Source: three-view drawing plus pictorial views. Frame: mm from the lowest corner of the part. A direction names the side the tool comes from. Coordinates: 2 decimals unless noted, no trailing zeros. Order: outer loops, then holes, each group sorted by start corner. A loop starts at its lowest first (then second) coordinate and runs counter-clockwise, first axis right, second up. Notation, with made-up numbers: M 23.5,60 L 73.5,60 A19 ccw 73.5,79 Z; hole C 11.5,22.25 d11. An arc over 180 degrees is marked long. One line per question, with ' | ' between items.
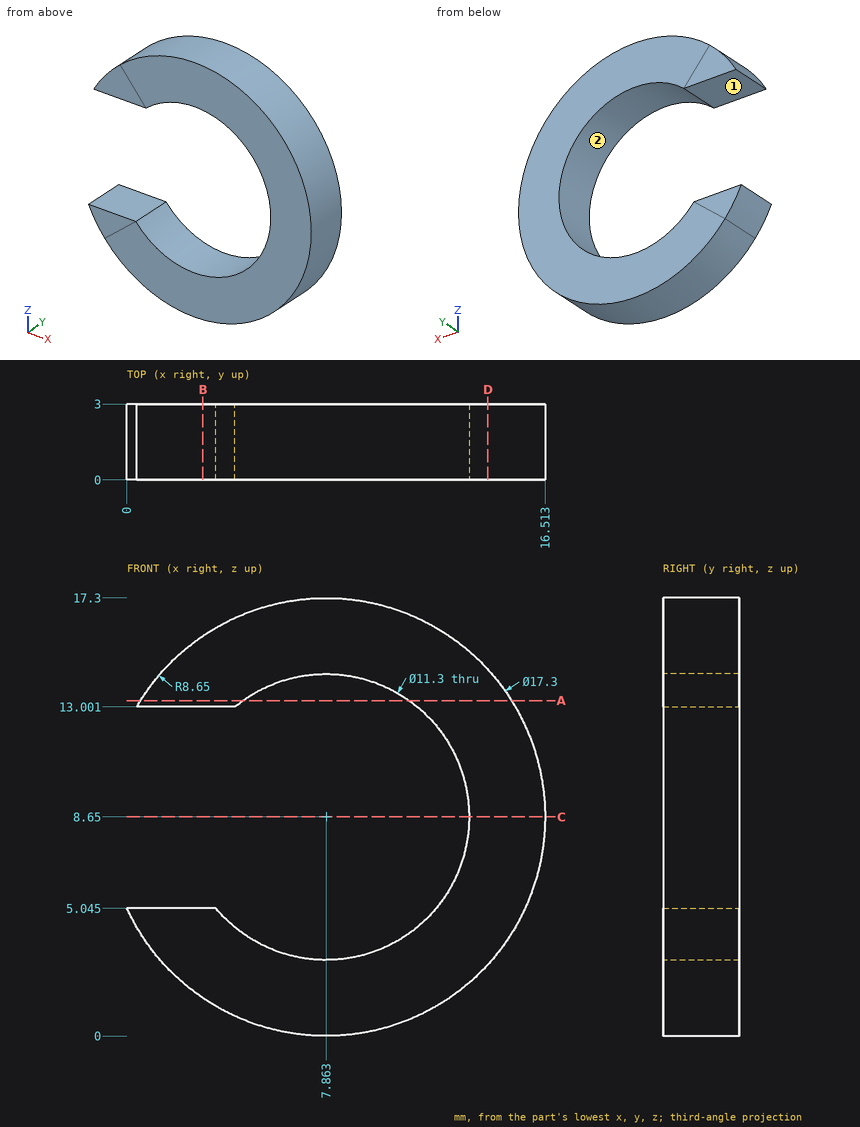
1. Pin query (flat end, axial travel): P1, Ø8, axis at x = 3.5, z = 11.5, coming from the +Y side. Return the tip coordinate at first contact, or that it passes through.
Response values:
P1: stops at y = 3
2. Material intervals for line 1 (Z direction, x = 8, y = 2.1); line 2 (X direction, y = 1.7, z = 8.65); line 3 (Z direction, x = 2.5, y = 2.6) (1 decimal), sorted ascending. Write a range as [from, to].
Response values:
line 1: z = [0, 3], [14.3, 17.3] | line 2: x = [13.51, 16.51] | line 3: z = [1.9, 5], [13, 15.4]
3. Section B-B, the plane x = 3. Output: boundary loops of the cut face in (y, z) (1 decimal).
Response values:
outline: M 0,1.5 L 3,1.5 L 3,5 L 0,5 Z; M 0,13 L 3,13 L 3,15.8 L 0,15.8 Z
4. Section C-C, the plane z = 8.65. Output: boundary loops of the cut face in (x, y).
Response values:
outline: M 13.51,0 L 16.51,0 L 16.51,3 L 13.51,3 Z
5. Access query for the marked faces 1 and 2. Directions: +Z, -Z, +X, -X, +Y, -Y. A direction counts if a zero-diameter tool reaches every point of the face in a straight line with its end or side. Return the directions, or none.
Response values:
face 1: -X, +Y, -Y | face 2: +Y, -Y
6. Section A-A, the plane z = 13.25. Output: boundary loops of the cut face in (x, y).
Response values:
outline: M 0.54,0 L 4.58,0 L 4.58,3 L 0.54,3 Z; M 11.14,0 L 15.19,0 L 15.19,3 L 11.14,3 Z
7. Section D-D, the plane x = 14.25. Output: boundary loops of the cut face in (y, z).
Response values:
outline: M 0,2.82 L 3,2.82 L 3,14.48 L 0,14.48 Z
